The model under review builds one solid part; all positions refer to its coordinate system, in mm. Face numbers are marked on the shaded views. A direction names the side the tool comes from. Round coordinates to 2 decimals unless told otherwise and drop trailing zeros. Answer as a JSON object with one key per item and string values. Group by question number.
1) The part is to be moulded in two halves that separate along X. For the marked faces 4, 5 and 6, say which applies: +X half, -X half, draft (parallel to the pull), parting line (faces both ways), or undercut.
2) To check wall thickness, follow line 1 (X direction, y = 0, z = -4.5); line 2 (Z direction, x = 31, y = 9); line 3 (Y direction, x = -7.5, z = 8.25). State the ranges of each line that lie inside material, in increasing order.
3) For the marked faces 1, 2 and 3, list the 3-axis set-ups (+Z, -Z, +X, -X, +Y, -Y) from which the entire face can be reached by the end or side of a thin tool; tool diameter is ignored.
4) Consider section A-A, the plane y = 0. Count the separate pieces of the cut face and the enclosed holes in it, then the cut area to 3 significant figures.
5) Insertion check: pin 1 Ø1.2 at (x, y) = (6, -20.5) entering from +Z; pin 2 Ø6.5 at (x, y) = (-42.5, 0) entering from +Z; pin 3 Ø15.5 at (x, y) = (0, 0) entering from -Z; pin 4 Ø5.5 at (x, y) = (28.5, -31) entering from -Z. Each pin has a flat end and moves straight along its axis. Give the tip position at first contact, or say it passes through.
Solid Edge part; units mm, degrees
sketch "Sketch1" plane through (60.3162, 60.3162, 0) normal (0, 0, 1) x (1, 0, 0)
  circle A0 centre (-60.3162, -60.3162) radius 50
  circle A1 centre (-60.3162, -60.3162) radius 7.5
extrude "Protrusion1" add sketch "Sketch1" along normal blind 6
sketch "Sketch2" plane through (0, 0, 0) normal (0, 0, -1) x (1, 0, 0)
  circle A0 centre (0, 0) radius 7.5
  circle A1 centre (0, 0) radius 12.5
extrude "Extrusionsausprägung_2" add sketch "Sketch2" along normal blind 8
chamfer "Fase_1" distance 0.5 angle 45 1 edges at (-12.5, 0, -8)
hole "Bohrung_1" at (-42.5, 0, 6) direction (0, 0, -1) diameter 4.5 end through all counterbore diameter 7 counterbore depth 4
pattern_circular "Pattern1" count 4 over 360 about axis through (0, 0, 6) along (0, 0, 1) of "Bohrung_1"
sketch "Sketch3" plane through (0, 0, 6) normal (0, 0, 1) x (-1, 0, 0)
  circle A0 centre (0, 0) radius 13
  circle A1 centre (0, 0) radius 24
extrude "Extrusionsausprägung_3" add sketch "Sketch3" along normal blind 11
chamfer "Fase_2" distance 0.5 angle 45 4 edges at (-50, 0, 6) (-50, 0, 0) (24, 0, 17) (13, 0, 17)
hole "Bohrung_2" at (-5.7884, -20.1865, 17) direction (0, 0, -1) diameter 2.459 depth 12 thread major 3 thread length 10
hole "Hole1" at (5.7884, -20.1865, 17) direction (0, 0, -1) diameter 2.459 depth 12 thread major 3 thread length 10
hole "Hole2" at (5.7884, 20.1865, 17) direction (0, 0, -1) diameter 2.459 depth 12 thread major 3 thread length 10
hole "Hole3" at (-5.7884, 20.1865, 17) direction (0, 0, -1) diameter 2.459 depth 12 thread major 3 thread length 10
hole "Bohrung_6" at (-30.052, 30.052, 0) direction (0, 0, 1) diameter 4.5 end up to next counterbore diameter 7 counterbore depth 4
pattern_circular "Pattern4" count 4 over 360 about axis through (0, 0, 0) along (0, 0, 1) of "Bohrung_6"
mirror "Mirror1" [suppressed]
sketch "Sketch4" plane through (0, 0, 6) normal (0, 0, 1) x (0, 1, 0)
  circle A0 centre (-42.5, 0) radius 2.25
  circle A1 centre (-42.5, 0) radius 4.5
extrude "Extrusionsausprägung_6" add sketch "Sketch4" against normal blind 6
properties material "Aluminium, 1060"
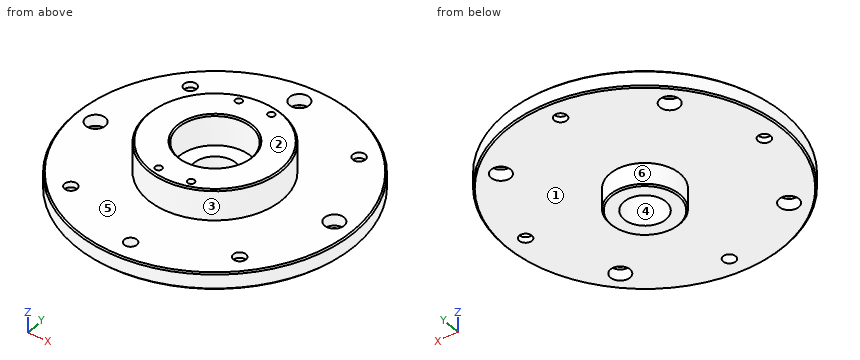
Results list:
{
 "1": {"face 4": "undercut", "face 5": "draft", "face 6": "parting line"},
 "2": {"line 1": "-12.5 to -7.5, 7.5 to 12.5", "line 2": "0 to 6", "line 3": "-22.8 to -10.62, 10.62 to 22.8"},
 "3": {"face 1": "-Z", "face 2": "+Z, +X, -X, +Y, -Y", "face 3": "+Z"},
 "4": {"separate pieces": "4", "enclosed holes": "0", "area": "757 mm^2"},
 "5": {"pin 1": "z = 5", "pin 2": "z = 2", "pin 3": "z = -8", "pin 4": "z = 0"}
}
